Verification items for the finished model (mm, model axes). Round coordinates to 2 decimals unless told otherwise and drop trailing zeros. Order: outer loops, then holes, each group sorted by start corner. A loop starts at its lowest first (then second) coordinate and runs counter-clockwise, first axis right, second up. Notation, with made-up numbers: M -33,8.25 L 18,8.25 A18 ccw 18,16.25 Z; hole C -34,66 d4. An arc over 180 degrees is marked long. Use CSV: the item, a comma, the result in double quotes. Start each with the question number.
Q1. Sectioned sample at C-C (z = 9.75). State how many separate pieces and enclosed holes the cut face has, and give its area (3 significant figures).
Q2. Sectioned sample at A-A (x = -27). Enter the section's corners in (y, z) (3 decimals).
Q3. Gauge pin test, flat ends, axial feed: pin 1 Ø3 at (x, y) = (77.88, -314.01) entering from -Z (3 decimals); pin 2 Ø4 at (x, y) = (-279, -209.5) entering from -Z. Record the tip position at first contact, or that the pin passes through.
Q4. Scan lines: line 1 (X direction, y = -204, z = 13); line 2 (Y direction, x = 38.1, z = 14.5) (3 decimals); line 3 (Y direction, x = 7.5, z = 1) (3 decimals). Record each from-to range of solid material in increasing order.
Q5. Sectioned sample at B-B (x = -168). Enter the section's corners in (y, z) (3 decimals), and give its area (3 significant figures).
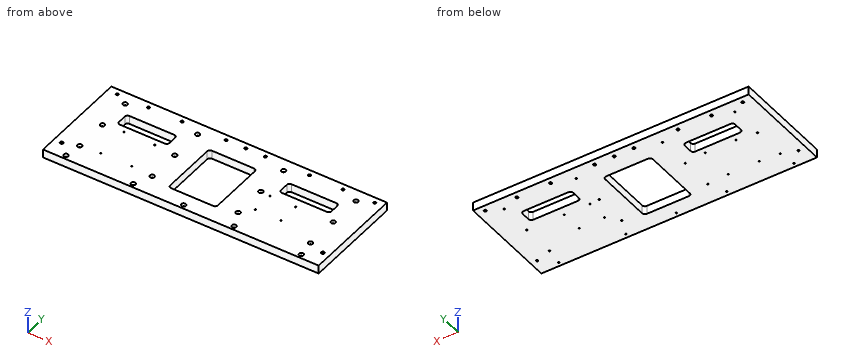
```python
from build123d import *

# Parameters (mm, degrees)
SKETCH1_W                                         = 624.84
SKETCH1_H                                         = 229.235
BOSS_EXTRUDE1_DEPTH                               = 19.05
F_5_64_0_07813_DIAMETER_HOLE1_D                   = 3.175
F_5_64_0_07813_DIAMETER_HOLE1_DEPTH               = 38.1
F_5_64_0_07813_DIAMETER_HOLE1_CSINK_D             = 10.16
F_5_64_0_07813_DIAMETER_HOLE1_CSINK_ANGLE         = 82
F_5_64_0_07813_DIAMETER_HOLE1_TIP                 = 0.953866233
F_15_64_0_23438_DIAMETER_HOLE1_D                  = 5.953252
F_15_64_0_23438_DIAMETER_HOLE1_DEPTH              = 19.05
F_2_CLEARANCE_HOLE1_D                             = 2.7051
F_2_CLEARANCE_HOLE1_DEPTH                         = 19.05
F_2_CLEARANCE_HOLE2_D                             = 2.7051
F_2_CLEARANCE_HOLE2_DEPTH                         = 19.05
CSK_FOR_6_FLAT_HEAD_MACHINE_SCREW_100_D           = 4.3053
CSK_FOR_6_FLAT_HEAD_MACHINE_SCREW_100_DEPTH       = 19.05
CSK_FOR_6_FLAT_HEAD_MACHINE_SCREW_100_CSINK_D     = 7.0866
CSK_FOR_6_FLAT_HEAD_MACHINE_SCREW_100_CSINK_ANGLE = 82
CUT_EXTRUDE2_REACH                                = 21.05
SKETCH18_W                                        = 114.3
SKETCH18_H                                        = 31.75
SKETCH18_W_2                                      = 107.95
SKETCH18_H_2                                      = 136.525
FILLET2_R                                         = 6.35


with BuildPart() as part:
    # Sketch1 → Boss-Extrude1 (new body)
    with BuildSketch(Plane.XY):
        with Locations((-183.67375, -247.3325)):
            Rectangle(SKETCH1_W, SKETCH1_H)
    extrude(amount=BOSS_EXTRUDE1_DEPTH)

    # 5/64 (0.07813) Diameter Hole1
    with Locations(Plane(origin=(-182.40375, -6471.459863233, 19.05), x_dir=(1, 0, 0), z_dir=(0, 0, 1))):
        with Locations((-262.8265, 6157.452363233), (-98.7933, 6157.452363233), (-262.8265, 6233.652363233), (-98.7933, 6233.652363233), (-262.8265, 6309.852363233), (-98.7933, 6309.852363233), (-267.97, 6119.034863233), (-115.57, 6119.034863233), (-1.27, 6119.034863233), (113.03, 6119.034863233), (265.43, 6119.034863233), (96.2533, 6309.852363233), (260.2865, 6309.852363233), (96.2533, 6233.652363233), (260.2865, 6233.652363233), (96.2533, 6157.452363233), (260.2865, 6157.452363233)):
            CounterSinkHole(F_5_64_0_07813_DIAMETER_HOLE1_D / 2, F_5_64_0_07813_DIAMETER_HOLE1_CSINK_D / 2, depth=F_5_64_0_07813_DIAMETER_HOLE1_DEPTH, counter_sink_angle=F_5_64_0_07813_DIAMETER_HOLE1_CSINK_ANGLE)
            with Locations((0, 0, -(F_5_64_0_07813_DIAMETER_HOLE1_DEPTH + F_5_64_0_07813_DIAMETER_HOLE1_TIP / 2))):  # 118° drill point
                Cone(0, F_5_64_0_07813_DIAMETER_HOLE1_D / 2, F_5_64_0_07813_DIAMETER_HOLE1_TIP, mode=Mode.SUBTRACT)

    # 15/64 (0.23438) Diameter Hole1
    with Locations(Plane(origin=(0, 0, 0), x_dir=(-1, 0, 0), z_dir=(0, 0, -1))):
        with Locations((402.9075, -146.05), (326.7075, -146.05), (226.85375, -146.05), (182.40375, -146.05), (137.95375, -146.05), (38.1, -146.05), (-38.1, -146.05), (473.86875, -146.05), (-110.1471, -146.05)):
            Hole(F_15_64_0_23438_DIAMETER_HOLE1_D / 2, depth=F_15_64_0_23438_DIAMETER_HOLE1_DEPTH)

    # #2 Clearance Hole1
    with Locations(Plane.XY.offset(19.05)):
        with Locations((-6.23545, -239.6), (-64.23545, -239.6), (-64.23545, -288.6), (-6.23545, -288.6)):
            Hole(F_2_CLEARANCE_HOLE1_D / 2, depth=F_2_CLEARANCE_HOLE1_DEPTH)

    # #2 Clearance Hole2
    with Locations(Plane(origin=(0, 0, 0), x_dir=(-1, 0, 0), z_dir=(0, 0, -1))):
        with Locations((399.72615, -233.172), (329.87615, -233.172), (329.87615, -310.642), (399.72615, -310.642)):
            Hole(F_2_CLEARANCE_HOLE2_D / 2, depth=F_2_CLEARANCE_HOLE2_DEPTH)

    # CSK for #6 Flat Head Machine Screw (100)1
    with Locations(Plane.XY.offset(19.05)):
        with Locations((113.823564524, -325.434443918), (-478.63125, -325.4375)):
            CounterSinkHole(CSK_FOR_6_FLAT_HEAD_MACHINE_SCREW_100_D / 2, CSK_FOR_6_FLAT_HEAD_MACHINE_SCREW_100_CSINK_D / 2, depth=CSK_FOR_6_FLAT_HEAD_MACHINE_SCREW_100_DEPTH, counter_sink_angle=CSK_FOR_6_FLAT_HEAD_MACHINE_SCREW_100_CSINK_ANGLE)

    # Sketch18 → Cut-Extrude2 (cut, up to next)
    with BuildSketch(Plane(origin=(0, 0, 0), x_dir=(-1, 0, 0), z_dir=(0, 0, -1)), mode=Mode.PRIVATE) as cut_extrude2_sk1:
        with Locations((0.00635, -203.2)):
            Rectangle(SKETCH18_W, SKETCH18_H)
    cut_extrude2_tool1 = extrude(cut_extrude2_sk1.sketch, amount=-CUT_EXTRUDE2_REACH, mode=Mode.PRIVATE) & part.part
    add(cut_extrude2_tool1.solids().sort_by_distance((-0.00635, -203.2, 0))[0], mode=Mode.SUBTRACT)
    # Sketch18 → Cut-Extrude2 (cut, up to next)
    with BuildSketch(Plane(origin=(0, 0, 0), x_dir=(-1, 0, 0), z_dir=(0, 0, -1)), mode=Mode.PRIVATE) as cut_extrude2_sk2:
        with Locations((367.34115, -203.2)):
            Rectangle(SKETCH18_W, SKETCH18_H)
    cut_extrude2_tool2 = extrude(cut_extrude2_sk2.sketch, amount=-CUT_EXTRUDE2_REACH, mode=Mode.PRIVATE) & part.part
    add(cut_extrude2_tool2.solids().sort_by_distance((-367.34115, -203.2, 0))[0], mode=Mode.SUBTRACT)
    # Sketch18 → Cut-Extrude2 (cut, up to next)
    with BuildSketch(Plane(origin=(0, 0, 0), x_dir=(-1, 0, 0), z_dir=(0, 0, -1)), mode=Mode.PRIVATE) as cut_extrude2_sk3:
        with Locations((183.67375, -255.5875)):
            Rectangle(SKETCH18_W_2, SKETCH18_H_2)
    cut_extrude2_tool3 = extrude(cut_extrude2_sk3.sketch, amount=-CUT_EXTRUDE2_REACH, mode=Mode.PRIVATE) & part.part
    add(cut_extrude2_tool3.solids().sort_by_distance((-183.67375, -255.5875, 0))[0], mode=Mode.SUBTRACT)

    # Fillet2
    fillet2_edges = [part.edges().sort_by_distance(p)[0] for p in [
        (57.14365, -219.075, 9.525),
        (57.14365, -187.325, 9.525),
        (-57.15635, -187.325, 9.525),
        (-57.15635, -219.075, 9.525),
        (-310.19115, -187.325, 9.525),
        (-424.49115, -187.325, 9.525),
        (-424.49115, -219.075, 9.525),
        (-310.19115, -219.075, 9.525),
        (-129.69875, -323.85, 9.525),
        (-129.69875, -187.325, 9.525),
        (-237.64875, -187.325, 9.525),
        (-237.64875, -323.85, 9.525),
    ]]
    fillet(fillet2_edges, radius=FILLET2_R)


solid = part.part
```
Verdict:
1,separate pieces,"1"
1,enclosed holes,"39"
1,area,"121,000 mm²"
2,outline,"M -361.95,0 L -219.075,0 L -219.075,19.05 L -361.95,19.05 Z; M -187.325,0 L -132.715,0 L -132.715,19.05 L -187.325,19.05 Z"
3,pin 1,"passes through"
3,pin 2,"stops at z = 0"
4,line 1,"x = -496.09 to -424.49, -310.19 to -237.65, -129.7 to -57.16, 57.14 to 128.75"
4,line 2,"y = -361.95 to -219.075, -187.325 to -149.027, -143.073 to -132.715"
4,line 3,"y = -361.95 to -219.075, -187.325 to -132.715"
5,outline,"M -361.95,0 L -323.85,0 L -323.85,19.05 L -361.95,19.05 Z; M -187.325,0 L -132.715,0 L -132.715,19.05 L -187.325,19.05 Z"
5,area,"1,770 mm²"
